```python
from build123d import *

# Parameters (mm, degrees)
SKETCH1_W           = 42
SKETCH1_H           = 42
BOSS_EXTRUDE1_DEPTH = 2.54
SKETCH2_W           = 42
SKETCH2_H           = 42
BOSS_EXTRUDE2_DEPTH = 9
SKETCH4_R           = 3.25
BOSS_EXTRUDE4_DEPTH = 42
SKETCH9_R           = 6.25
SKETCH9_R_2         = 2.05
BOSS_EXTRUDE5_DEPTH = 6.5
SKETCH10_R          = 2.05
CUT_EXTRUDE1_DEPTH  = 8
SKETCH12_W          = 17.78
SKETCH12_H          = 2
CUT_EXTRUDE2_DEPTH  = 4
FILLET1_R           = 3


with BuildPart() as part:
    # Sketch1 → Boss-Extrude1 (new body)
    with BuildSketch(Plane(origin=(0, 0, 0), x_dir=(1, 0, 0), z_dir=(0, 1, 0))):
        Rectangle(SKETCH1_W, SKETCH1_H)
    extrude(amount=BOSS_EXTRUDE1_DEPTH)

    # Sketch2 → Boss-Extrude2 (add)
    with BuildSketch(Plane(origin=(0, 2.54, 0), x_dir=(1, 0, 0), z_dir=(0, 1, 0))):
        Rectangle(SKETCH2_W, SKETCH2_H)
        with BuildLine():
            Line((-17, 11.522774425), (-17, -11.522774425))
            ThreePointArc((-17, -11.522774425), (-16.869274473, -11.859874356), (-16.545454545, -12.020704023))
            ThreePointArc((-16.545454545, -12.020704023), (-13.464466094, -13.464466094), (-12.020704023, -16.545454545))
            ThreePointArc((-12.020704023, -16.545454545), (-11.859874356, -16.869274473), (-11.522774425, -17))
            Line((-11.522774425, -17), (11.522774425, -17))
            ThreePointArc((11.522774425, -17), (11.859874356, -16.869274473), (12.020704023, -16.545454545))
            ThreePointArc((12.020704023, -16.545454545), (13.464466094, -13.464466094), (16.545454545, -12.020704023))
            ThreePointArc((16.545454545, -12.020704023), (16.869274473, -11.859874356), (17, -11.522774425))
            Line((17, -11.522774425), (17, 11.522774425))
            ThreePointArc((17, 11.522774425), (16.869274473, 11.859874356), (16.545454545, 12.020704023))
            ThreePointArc((16.545454545, 12.020704023), (13.464466094, 13.464466094), (12.020704023, 16.545454545))
            ThreePointArc((12.020704023, 16.545454545), (11.859874356, 16.869274473), (11.522774425, 17))
            Line((11.522774425, 17), (-11.522774425, 17))
            ThreePointArc((-11.522774425, 17), (-11.859874356, 16.869274473), (-12.020704023, 16.545454545))
            ThreePointArc((-12.020704023, 16.545454545), (-13.464466094, 13.464466094), (-16.545454545, 12.020704023))
            ThreePointArc((-16.545454545, 12.020704023), (-16.869274473, 11.859874356), (-17, 11.522774425))
        make_face(mode=Mode.SUBTRACT)
    extrude(amount=BOSS_EXTRUDE2_DEPTH)

    # Sketch4 → Boss-Extrude4 (add)
    with BuildSketch(Plane.ZY.offset(21)):
        with BuildLine():
            Line((7.5, 0), (5.927131841, -10))
            ThreePointArc((5.927131841, -10), (0, -15.067740305), (-5.927131841, -10))
            Line((-5.927131841, -10), (-7.5, 0))
            Line((-7.5, 0), (7.5, 0))
        make_face()
        with Locations((0, -9.067740305)):
            Circle(SKETCH4_R, mode=Mode.SUBTRACT)
    extrude(amount=-BOSS_EXTRUDE4_DEPTH)

    # Sketch9 → Boss-Extrude5 (add)
    with BuildSketch(Plane(origin=(0, 2.54, 0), x_dir=(1, 0, 0), z_dir=(0, 1, 0))):
        with Locations((8, 0)):
            Circle(SKETCH9_R)
        with Locations((8, 0)):
            Circle(SKETCH9_R_2, mode=Mode.SUBTRACT)
        with Locations((-8, 0)):
            Circle(SKETCH9_R)
        with Locations((-8, 0)):
            Circle(SKETCH9_R_2, mode=Mode.SUBTRACT)
    extrude(amount=BOSS_EXTRUDE5_DEPTH)

    # Sketch10 → Cut-Extrude1 (cut)
    with BuildSketch(Plane(origin=(0, 11.54, 0), x_dir=(1, 0, 0), z_dir=(0, 1, 0))):
        with Locations((-17, 17)):
            Circle(SKETCH10_R)
        with Locations((17, 17)):
            Circle(SKETCH10_R)
        with Locations((-17, -17)):
            Circle(SKETCH10_R)
        with Locations((17, -17)):
            Circle(SKETCH10_R)
    extrude(amount=-CUT_EXTRUDE1_DEPTH, mode=Mode.SUBTRACT)

    # Sketch12 → Cut-Extrude2 (cut)
    with BuildSketch(Plane(origin=(0, 0, -21), x_dir=(-1, 0, 0), z_dir=(0, 0, -1))):
        with Locations((0, 10.54)):
            Rectangle(SKETCH12_W, SKETCH12_H)
    extrude(amount=-CUT_EXTRUDE2_DEPTH, mode=Mode.SUBTRACT)

    # Fillet1
    fillet1_edges = [part.edges().sort_by_distance(p)[0] for p in [
        (21, 5.77, 21),
        (-21, 5.77, 21),
        (-21, 5.77, -21),
        (21, 5.77, -21),
    ]]
    fillet(fillet1_edges, radius=FILLET1_R)


solid = part.part
```
Source: CAD feature listing. Evaluate the final solid. Frame: model axes, mm. A direction names the side the tool comes from. Round coordinates to 2 decimals unless told otherwise and drop trailing zeros. Loops run counter-clockwise (first coordinate to the right, second up) from the corner with the lowest first, then second, coordinate; pieces in that order, holes last.
1. Section query C-C on x = 8. Output: boundary loops of the cut face in (y, z).
2. Contact query for flat-ended pins moving along their axis: pin 1 (7 mm diameter, centred on x = 6, z = -16.5, fed in from -Y); pin 2 (2 mm diameter, centred on x = 1, z = -18.5, fed in from +Y); pin 3 (4 mm diameter, centred on y = -9.07, z = 0, fed in from -X); pin 4 (4.5 mm diameter, centred on x = 17.5, z = 17, fed in from +Y). Output: stop coordinate, or through.
3. Mould query, pull axis Z, two halves, no side actions, for faces 4 (the cylindrical face through (-20.14, 5.85, 20.1)), 5 (the flat face through (0, 9.54, -19)), 6 (the cylindrical face through (5.95, 5.74, -0.09)), 7 (the flat face through (-0.294, -5.07, -6.703)). Classes: released by +Z, released by -Z, zero draft, split by the parting line, or undercut.
4. Ray query, L1, parallel to X at y = 4.5, z = 0; L2, parallel to Z at x = -8, y = 7.25; L3, parallel to X at y = 9.25, z = 2.5. Return the intervals inside material, ascending.
5. Section query B-B on z = 0. Output: boundary loops of the cut face in (x, y).
6. Section query A-A on y = 6.5. Give the number of separate pieces and of enclosed holes in the cut face, and give its area (3 significant figures).
7. Access query for faces 1 (the cylindrical face through (-20.14, 5.69, -20.1)), 2 (the flat face through (-8.89, 11, -19)), 3 (the flat face through (-17, 7, 0)). Directions: +Z, -Z, +X, -X, +Y, -Y. A direction counts if a zero-diameter tool reaches every point of the face in a straight line with its end or side. Return the directions, or none.
Answers below:
1. outline: (-10, -5.93) - (0, -7.5) - (0, -21) - (9.54, -21) - (9.54, -17) - (2.54, -17) - (2.54, -6.25) - (9.04, -6.25) - (9.04, -2.05) - (2.54, -2.05) - (2.54, 2.05) - (9.04, 2.05) - (9.04, 6.25) - (2.54, 6.25) - (2.54, 17) - (11.54, 17) - (11.54, 21) - (0, 21) - (0, 7.5) - (-10, 5.93) arc R6 ccw to start; hole circle Ø6.5 at (-9.07, 0)
2. pin 1: stops at y = 0
2. pin 2: stops at y = 9.54
2. pin 3: passes through
2. pin 4: stops at y = 11.54
3. face 4: released by +Z
3. face 5: zero draft
3. face 6: undercut
3. face 7: released by -Z
4. L1: x = -21 to -17, -14.25 to -10.05, -5.95 to -1.75, 1.75 to 5.95, 10.05 to 14.25, 17 to 21
4. L2: z = -21 to -17, -6.25 to -2.05, 2.05 to 6.25, 17 to 21
4. L3: x = -21 to -17, 17 to 21
5. outline: (-21, -15.07) - (21, -15.07) - (21, -12.32) - (-21, -12.32) - close; (-21, -5.82) - (21, -5.82) - (21, 11.54) - (17, 11.54) - (17, 2.54) - (14.25, 2.54) - (14.25, 9.04) - (10.05, 9.04) - (10.05, 2.54) - (5.95, 2.54) - (5.95, 9.04) - (1.75, 9.04) - (1.75, 2.54) - (-1.75, 2.54) - (-1.75, 9.04) - (-5.95, 9.04) - (-5.95, 2.54) - (-10.05, 2.54) - (-10.05, 9.04) - (-14.25, 9.04) - (-14.25, 2.54) - (-17, 2.54) - (-17, 11.54) - (-21, 11.54) - close
6. separate pieces: 3
6. enclosed holes: 7
6. area: 845 mm2
7. face 1: -Z, -X, +Y, -Y
7. face 2: -Z, +Y
7. face 3: +Y
